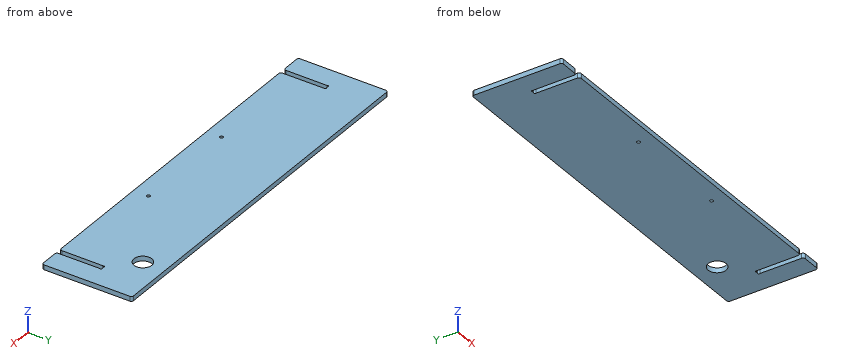
from build123d import *

# Parameters (mm, degrees)
ESQUISSE1_W         = 590.5
ESQUISSE1_H         = 280.25
BOSS_EXTRUDE1_DEPTH = 15
CUT_EXTRUDE1_DEPTH  = 654.800667253
ESQUISSE3_R         = 5
CUT_EXTRUDE2_DEPTH  = 654.800667253
CONG_1_R            = 7
SKETCH1_R           = 28
CUT_EXTRUDE3_DEPTH  = 1214.888818014


with BuildPart() as part:
    # Esquisse1 → Boss-Extrude1 (new body)
    with BuildSketch(Plane.XY):
        with Locations((295.25, 140.125)):
            Rectangle(ESQUISSE1_W, ESQUISSE1_H)
    extrude(amount=BOSS_EXTRUDE1_DEPTH)

    # Esquisse2 → Cut-Extrude1 (cut, through all)
    with BuildSketch(Plane.XY.offset(15)):
        with BuildLine():
            Line((70.977649355, 140.125), (76.647350645, 140.125))
            ThreePointArc((76.647350645, 140.125), (76.980108702, 140.181987765), (77.274940482, 140.346455848))
            ThreePointArc((77.274940482, 140.346455848), (81.406698158, 140.130786526), (81.644207297, 136.00022674))
            ThreePointArc((81.644207297, 136.00022674), (81.481699427, 135.705678195), (81.426062442, 135.373906919))
            Line((81.426062442, 135.373906919), (81.8125, 0))
            Line((81.8125, 0), (65.8125, 0))
            Line((65.8125, 0), (66.198937558, 135.373906919))
            ThreePointArc((66.198937558, 135.373906919), (66.143300573, 135.705678195), (65.980792703, 136.00022674))
            ThreePointArc((65.980792703, 136.00022674), (66.218301842, 140.130786526), (70.350059518, 140.346455848))
            ThreePointArc((70.350059518, 140.346455848), (70.644891298, 140.181987765), (70.977649355, 140.125))
        make_face()
    extrude(amount=-CUT_EXTRUDE1_DEPTH, mode=Mode.SUBTRACT)

    # Esquisse3 → Cut-Extrude2 (cut, through all)
    with BuildSketch(Plane.XY.offset(15)):
        with Locations((422.0625, 46.708333333)):
            Circle(ESQUISSE3_R)
    extrude(amount=-CUT_EXTRUDE2_DEPTH, mode=Mode.SUBTRACT)

    # Cong_1
    cong_1_edges = [part.edges().sort_by_distance(p)[0] for p in [
        (81.8125, 0, 7.5),
        (65.8125, 0, 7.5),
        (0, 280.25, 7.5),
        (0, 0, 7.5),
    ]]
    fillet(cong_1_edges, radius=CONG_1_R)

    # Sym_trie1: part across plane


with BuildPart() as part_1:
    add(part.part)
    add(part.part.mirror(Plane(origin=(590.5, 0, 15), x_dir=(0, 0, 1), z_dir=(-1, 0, 0))))

    # Sketch1 → Cut-Extrude3 (cut, through all)
    with BuildSketch(Plane.XY.offset(15)):
        with Locations((1027.1875, 210.25)):
            Circle(SKETCH1_R)
    extrude(amount=-CUT_EXTRUDE3_DEPTH, mode=Mode.SUBTRACT)


solid = part_1.part
Geometry: final body of the model. Coordinates: model frame, mm. Give positions to 0.01 mm unless a question says otherwise; leave off trailing zeros. Order: outer loops, then holes, each group sorted by start corner. A loop starts at its lowest first (then second) coordinate and runs counter-clockwise, first axis right, second up. Notation, with made-up numbers: (4, 47) - (62, 47) arc R18 ccw to (62, 78) - close; hole circle Ø9 at (-4.75, -20). An arc over 180 degrees is marked (long way). Use CSV: the item, a comma, the result in double quotes.
1. Material intervals for line 1 along X through (y, z) = (96, 5.75); line 2 along X through (y, z) = (123, 13); line 3 along X through (y, z) = (199, 4.5), sorted ascending. Write a range as from..to.
Answers below:
line 1,"0..66.09, 81.54..1099.46, 1114.91..1181"
line 2,"0..66.16, 81.46..1099.54, 1114.84..1181"
line 3,"0..1001.55, 1052.83..1181"
2. Section query A-A (y = 210.25). Output: boundary loops of the cut face in (x, z).
Answers below:
outline,"(0, 0) - (999.19, 0) - (999.19, 15) - (0, 15) - close; (1055.19, 0) - (1181, 0) - (1181, 15) - (1055.19, 15) - close"
3. Section query B-B (y = 107.5). Output: boundary loops of the cut face in (x, z).
Answers below:
outline,"(0, 0) - (66.12, 0) - (66.12, 15) - (0, 15) - close; (81.51, 0) - (1099.49, 0) - (1099.49, 15) - (81.51, 15) - close; (1114.88, 0) - (1181, 0) - (1181, 15) - (1114.88, 15) - close"
4. Contact query for flat-ended pins moving along their axis: pin 1 (3 mm diameter, centred on x = 1108.5, z = 7.5, fed in from -Y) (3 decimals); pin 2 (6 mm diameter, centred on x = 422.06, y = 46.71, fed in from +Z). Output: stop coordinate, or through.
Answers below:
pin 1,"y = 140.125"
pin 2,"through"
5. Section query C-C (z = 9.5). Give the number of separate pieces and of enclosed holes in the cut face, plus the area to 3 significant figures.
Answers below:
separate pieces,"1"
enclosed holes,"3"
area,"324,000 mm2"
